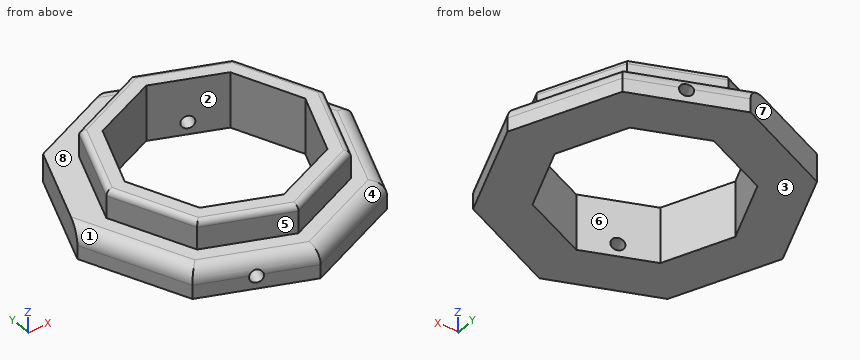
from build123d import *

# Parameters (mm, degrees)
F1_DEPTH     = 10
F3_DEPTH     = 10
F5_DEPTH     = 23.6474
F6_R         = 2.25
F7_DEPTH     = 107.696
F8_R         = 2
F9_T1_DEPTH  = 63.6683432365
F9_T3_DEPTH  = 63.6683432365
F9_T5_DEPTH  = 63.6683432365
F9_T7_DEPTH  = 63.6683432365
F9_T9_DEPTH  = 63.6683432365
F9_T11_DEPTH = 63.6683432365


# Not quite as in the source:
# - a fillet or chamfer that OpenCascade refuses, or shapes differently, is made with other operations: its cross-section is extruded or revolved along the edge and cut away or added


with BuildPart() as f1:
    # F0 (on Top) → F1 (new body)
    with BuildSketch(Plane.XY):
        Polygon((50, 0), (35.3553390593, 35.3553390593), (0, 50), (-35.3553390593, 35.3553390593), (-50, 0), (-35.3553390593, -35.3553390593), (0, -50), (35.3553390593, -35.3553390593), align=None)
    extrude(amount=-F1_DEPTH)

    # F2 (on face) → F3 (join)
    with BuildSketch(Plane.XY):
        Polygon((-27.9307178569, -27.9307178569), (0, -39.5), (27.9307178569, -27.9307178569), (39.5, 0), (27.9307178569, 27.9307178569), (0, 39.5), (-27.9307178569, 27.9307178569), (-39.5, 0), align=None)
    extrude(amount=F3_DEPTH)

    # F4 (on face) → F5 (cut)
    with BuildSketch(Plane.XY.offset(10)):
        Polygon((-32.7123950097, 0.1427250341), (-23.2320781797, -23.0302345008), (-0.1427250341, -32.7123950097), (23.0302345008, -23.2320781797), (32.7123950097, -0.1427250341), (23.2320781797, 23.0302345008), (0.1427250341, 32.7123950097), (-23.0302345008, 23.2320781797), align=None)
    extrude(amount=-F5_DEPTH, mode=Mode.SUBTRACT)

    # F6 (on face) → F7 (cut)
    with BuildSketch(Plane(origin=(17.6776695297, 42.6776695297, 0), x_dir=(-0.9238795325, 0.3826834324, 0), z_dir=(0.3826834324, 0.9238795325, 0))):
        with Locations((0, -5.5711902678)):
            Circle(F6_R)
    extrude(amount=-F7_DEPTH, mode=Mode.SUBTRACT)

    # F8
    f8_edges = [f1.edges().sort_by_distance(p)[0] for p in [
        (33.715359, 13.965359, 10),
        (33.715359, -13.965359, 10),
        (13.965359, -33.715359, 10),
        (-13.965359, -33.715359, 10),
        (-33.715359, -13.965359, 10),
        (-33.715359, 13.965359, 10),
        (-13.965359, 33.715359, 10),
        (13.965359, 33.715359, 10),
    ]]
    fillet(f8_edges, radius=F8_R)

    # F9: fillet of radius 5.08 on 6 edges, made by hand

    # F9_s2 → F9_t1 (cut)
    with BuildSketch(Plane(origin=(-12.1824100614, -29.4109395926, 0), x_dir=(0, 0, 1), z_dir=(0.3826834324, 0.9238795325, 0))):
        with BuildLine():
            ThreePointArc((0, 41.1139766256), (-1.4878975516, 44.706079074), (-5.08, 46.1939766256))
            Line((-5.08, 46.1939766256), (0, 46.1939766256))
            Line((0, 46.1939766256), (0, 41.1139766256))
        make_face()
    extrude(amount=F9_T1_DEPTH, mode=Mode.SUBTRACT)

    # F9_s4 → F9_t3 (cut)
    with BuildSketch(Plane(origin=(-29.4109395926, -12.1824100614, 0), x_dir=(0, 0, 1), z_dir=(0.9238795325, 0.3826834324, 0))):
        with BuildLine():
            ThreePointArc((0, 41.1139766256), (-1.4878975516, 44.706079074), (-5.08, 46.1939766256))
            Line((-5.08, 46.1939766256), (0, 46.1939766256))
            Line((0, 46.1939766256), (0, 41.1139766256))
        make_face()
    extrude(amount=F9_T3_DEPTH, mode=Mode.SUBTRACT)

    # F9_s6 → F9_t5 (cut)
    with BuildSketch(Plane(origin=(-29.4109395926, 12.1824100614, 0), x_dir=(0, 0, 1), z_dir=(0.9238795325, -0.3826834324, 0))):
        with BuildLine():
            ThreePointArc((0, 41.1139766256), (-1.4878975516, 44.706079074), (-5.08, 46.1939766256))
            Line((-5.08, 46.1939766256), (0, 46.1939766256))
            Line((0, 46.1939766256), (0, 41.1139766256))
        make_face()
    extrude(amount=F9_T5_DEPTH, mode=Mode.SUBTRACT)

    # F9_s8 → F9_t7 (cut)
    with BuildSketch(Plane(origin=(12.1824100614, -29.4109395926, 0), x_dir=(0, 0, 1), z_dir=(-0.3826834324, 0.9238795325, 0))):
        with BuildLine():
            ThreePointArc((0, 41.1139766256), (-1.4878975516, 44.706079074), (-5.08, 46.1939766256))
            Line((-5.08, 46.1939766256), (0, 46.1939766256))
            Line((0, 46.1939766256), (0, 41.1139766256))
        make_face()
    extrude(amount=F9_T7_DEPTH, mode=Mode.SUBTRACT)

    # F9_s10 → F9_t9 (cut)
    with BuildSketch(Plane(origin=(-12.1824100614, 29.4109395926, 0), x_dir=(0, 0, 1), z_dir=(0.3826834324, -0.9238795325, 0))):
        with BuildLine():
            ThreePointArc((0, 41.1139766256), (-1.4878975516, 44.706079074), (-5.08, 46.1939766256))
            Line((-5.08, 46.1939766256), (0, 46.1939766256))
            Line((0, 46.1939766256), (0, 41.1139766256))
        make_face()
    extrude(amount=F9_T9_DEPTH, mode=Mode.SUBTRACT)

    # F9_s12 → F9_t11 (cut)
    with BuildSketch(Plane(origin=(29.4109395926, -12.1824100614, 0), x_dir=(0, 0, 1), z_dir=(-0.9238795325, 0.3826834324, 0))):
        with BuildLine():
            ThreePointArc((0, 41.1139766256), (-1.4878975516, 44.706079074), (-5.08, 46.1939766256))
            Line((-5.08, 46.1939766256), (0, 46.1939766256))
            Line((0, 46.1939766256), (0, 41.1139766256))
        make_face()
    extrude(amount=F9_T11_DEPTH, mode=Mode.SUBTRACT)


solid = f1.part
Can you work these out from the model? Positions are in its coordinate system, mm. Face numbers are marked on the shaded views. A direction names the side the tool comes from. Give positions to 0.01 mm unless a question says otherwise; leave off trailing zeros. Write each loop counter-clockwise with the first axis right and the second up, starting at its lowest first coordinate (ties: lowest second). Pieces come first, ordered by that corner, then holes. Notation, with made-up numbers: M 37,69 L 47,69 A9 cw 47,79 Z; hole C -23.75,48.25 d8. An arc over 180 degrees is marked long. Answer in a Markdown table with one row per item. Add a question column.
Item 1: We'd pull the mould along Y, two halves only. Please class the marked faces 1, 2 and 3: released by +Y, released by -Y, zero draft, split by the parting line, or undercut.
Item 2: For pin 1 Ø12 at (x, z) = (8.5, 6.5) entering from +Y; pin 2 Ø6 at (x, z) = (6, 2) entering from -Y; pin 3 Ø12 at (x, y) = (33, 14) entering from +Z; pin 4 Ø12 at (y, z) = (24, -5.5) entering from -X, each with a flat end and sliding along its axis, tell me the tip position at first contact or that it passes through.
Item 3: Imagine slicing it at A-A, the plane z = 2.5. Write out the boundary of the cut face in (x, y).
Item 4: On a 3-axis mill with a long thin cutter (end or side, diameter ignored), from which of +Z, -Z, +X, -X, +Y, -Y can I reach the whole of each face in a straight line? I mean the marked faces 4, 5, 6, 7 and 8. Say none if no direction works.
Item 5: Please list where these lines run through material, in increasing order: L1, parallel to X at y = -30.5, z = -5.5; L2, parallel to Z at x = -9.5, y = 40; L3, parallel to Y at x = -31.5, z = -2.75.
Evaluation:
| question | item | result |
|---|---|---|
| 1 | face 1 | released by -Y |
| 1 | face 2 | undercut |
| 1 | face 3 | zero draft |
| 2 | pin 1 | stops at y = 38.46 |
| 2 | pin 2 | stops at y = -45.46 |
| 2 | pin 3 | stops at z = 10 |
| 2 | pin 4 | stops at x = -42.54 |
| 3 | outline | M -39.5,0 L -27.93,-27.93 L 0,-39.5 L 27.93,-27.93 L 39.5,0 L 27.93,27.93 L 0,39.5 L -27.93,27.93 Z; hole M -32.71,0.14 L -23.23,-23.03 L -0.14,-32.71 L 23.03,-23.23 L 32.71,-0.14 L 23.23,23.03 L 0.14,32.71 L -23.03,23.23 Z |
| 4 | face 4 | +Z, +X, -Y |
| 4 | face 5 | +Z, -X, -Y |
| 4 | face 6 | +Z, -Z |
| 4 | face 7 | +Z, -Z, -X, +Y |
| 4 | face 8 | +Z |
| 5 | L1 | x = -37.37 to -15.07, -10.2 to -5.42, 5.27 to 37.37 |
| 5 | L2 | z = -10 to 0 |
| 5 | L3 | y = -36.34 to -2.82, 3.03 to 36.95 |
